The listing builds one solid part. Answer for the finished solid, in the listing's coordinates (mm). Face numbers are marked on the shaded views. Coordinates: 2 decimals unless noted, no trailing zeros. Order: outer loops, then holes, each group sorted by start corner. A loop starts at its lowest first (then second) coordinate and runs counter-clockwise, first axis right, second up. Notation, with made-up numbers: (-18, 84.5) -> (22, 84.5) arc R13 cw to (22, 91.5) -> close; hole circle Ø6 at (66.5, -21.75). An arc over 180 degrees is marked (long way). Return JSON: item names as keys, results as strings.
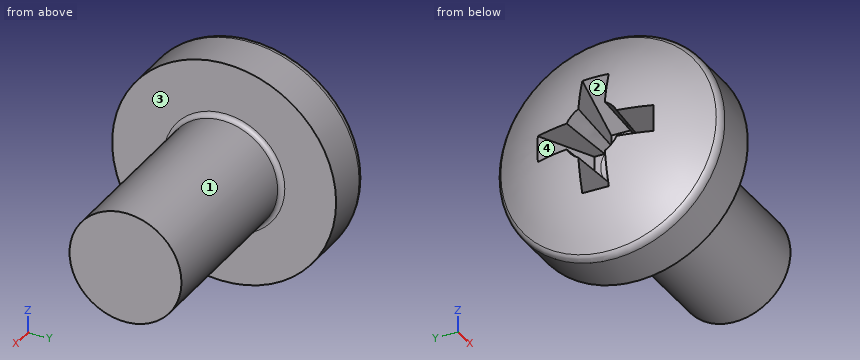
from build123d import *

# Parameters (mm, degrees)
RECPAT_COUNT = 2
RECPAT_ANGLE = 90


with BuildPart() as part:
    # Fillet1: read off the stored shape, not the designer's step
    # Fillet1 outline → Fillet1 (revolve)
    with BuildSketch(Plane.YX):
        with BuildLine():
            Line((3, 4.85), (3, 14.6))
            Line((3, 14.6), (0, 14.6))
            Line((0, 14.6), (0, 0))
            ThreePointArc((0, 0), (3.027985079, 0.469454036), (5.771670194, 1.833738728))
            ThreePointArc((5.771670194, 1.833738728), (5.939532013, 2.026424569), (6, 2.274716834))
            Line((6, 2.274716834), (6, 4.6))
            Line((6, 4.6), (3.25, 4.6))
            ThreePointArc((3.25, 4.6), (3.073223305, 4.673223305), (3, 4.85))
        make_face()
    revolve(axis=Axis((0, 0, 0), (1, 0, 0)))

    # Sketch3 → Recess section 0
    with BuildSketch(Plane(origin=(0, 0, 0), x_dir=(0, 0, -1), z_dir=(1, 0, 0))):
        with BuildLine():
            Line((0.71, -3.35), (-0.71, -3.35))
            Line((-0.71, -3.35), (-0.71, 3.35))
            Line((-0.71, 3.35), (0.71, 3.35))
            Line((0.71, 3.35), (0.71, -3.35))
        make_face()
    # Sketch4 → Recess section 1
    with BuildSketch(Plane(origin=(3.46, 0, 0), x_dir=(0, 0, -1), z_dir=(1, 0, 0))):
        with BuildLine():
            Line((0.71, -1.624907925), (-0.71, -1.624907925))
            Line((-0.71, -1.624907925), (-0.71, 1.624907925))
            Line((-0.71, 1.624907925), (0.71, 1.624907925))
            Line((0.71, 1.624907925), (0.71, -1.624907925))
        make_face()
    recess = loft(mode=Mode.SUBTRACT)

    # RecPat: Recess ×2 about axis
    recpat_axis = Axis((0, 0, 0), (1, 0, 0))
    for i in range(1, RECPAT_COUNT):
        add(recess.rotate(recpat_axis, i * RECPAT_ANGLE / (RECPAT_COUNT - 1)), mode=Mode.SUBTRACT)

    # RecCorSke → RecessCore (revolve, cut)
    with BuildSketch(Plane.XY, mode=Mode.PRIVATE) as recesscore_sk:
        Polygon((0, 0), (0, 1.522446769), (3.46, 1.2805), (3.876059671, 0), align=None)
    revolve(recesscore_sk.sketch.rotate(Axis((-3.175, 0, 0), (1, 0, 0)), 90), axis=Axis((-3.175, 0, 0), (1, 0, 0)), mode=Mode.SUBTRACT)


solid = part.part
1. Each of these flat-tipped pins is pushed along its axis until it touches: pin 1 Ø4 at (y, z) = (-3.5, 1.5) entering from -X; pin 2 Ø1 at (y, z) = (-4, -1.5) entering from +X; pin 3 Ø2 at (x, y) = (6, 0) entering from -Z; pin 4 Ø0.6 at (y, z) = (-0.5, 1.5) entering from -X. Where does it stop, or does it pass through?
Answer block:
{"pin 1": "stops at x = 0.16", "pin 2": "stops at x = 4.6", "pin 3": "stops at z = -3", "pin 4": "stops at x = 0.12"}
2. The part is cut by section A-A on x = 13.25. Give the vertices of the cut face in (y, z), and give its area (3 significant figures).
Answer block:
{"outline": "circle Ø6 at (0, 0)", "area": "28.3 mm2"}
3. Determine the mould class of the marked faces 1, 2, 3 and 4 for opening direction Z: pulls with the +Z half, pulls with the -Z half, needs draft (parallel to the pull), parting line crosses it, or undercut.
Answer block:
{"face 1": "parting line crosses it", "face 2": "undercut", "face 3": "needs draft", "face 4": "undercut"}
4. Consider line 1 (Z direction, x = 1.5, y = 0.75); line 2 (Z direction, x = 2, y = -1.25); line 3 (X direction, y = -4.25, z = -3). Determine where each line is inside the solid, lowest interval first. Write a range as from..to.
Answer block:
{"line 1": "z = -5.21..-1.2, 1.2..5.21", "line 2": "z = -5.79..-0.71, 0.71..5.79", "line 3": "x = 1.46..4.6"}
